```python
from build123d import *

# Parameters (mm, degrees)
EXTRUDE_1_DEPTH     = 8
CUT_EXTRUDE_1_DEPTH = 3


with BuildPart() as part:
    # Эскиз2 → Бобышка-Вытянуть1 (new body)
    with BuildSketch(Plane.XY):
        Polygon((0, 0), (40, 0), (40, 10), (27.5, 12), (27.5, 22), (42.5, 35), (42.5, 55), (-2.5, 55), (-2.5, 35), (12.5, 22), (12.5, 12), (0, 10), align=None)
    extrude(amount=EXTRUDE_1_DEPTH)

    # Эскиз3 → Вырез-Вытянуть1 (cut)
    with BuildSketch(Plane(origin=(0, 0, 0), x_dir=(-1, 0, 0), z_dir=(0, 0, -1))):
        Polygon((-40, 10), (-27.5, 12), (-27.5, 22), (-42.5, 35), (2.5, 35), (-12.5, 22), (-12.5, 12), (0, 10), align=None)
    extrude(amount=-CUT_EXTRUDE_1_DEPTH, mode=Mode.SUBTRACT)


solid = part.part
```
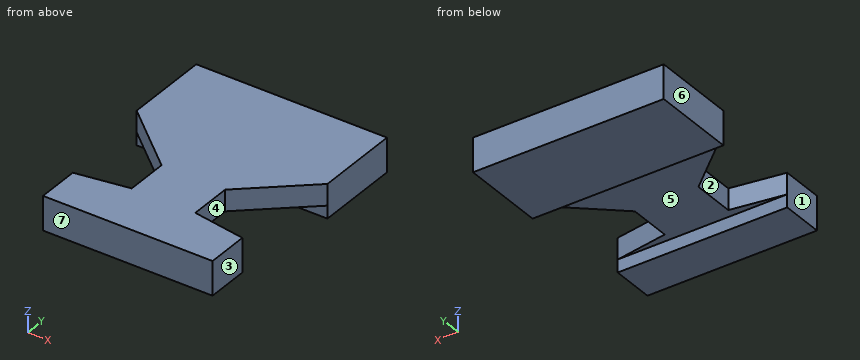
Input: part model. Units: mm. Frame: model coordinates. Face numbers are marked on the shaded views. A direction names the side the tool comes from. Coordinates: 2 decimals unless noted, no trailing zeros. Write each loop counter-clockwise with the first axis right and the second up, starting at its lowest first coordinate (ties: lowest second). Pieces come first, ordered by that corner, then holes.
1) Set-up query: the marked faces 1, 2 and 3. Return all of +Z, -Z, +X, -X, +Y, -Y with unobstructed straight access to the full face (end or side cutting, diameter ignored); none if empty.
2) Mould query, pull axis Y, two halves, no side actions, for the marked faces 4, 5, 6 and 7. Classes: pulls with the +Y half, pulls with the -Y half, needs draft (parallel to the pull), parting line crosses it, or undercut.
3) Pin query (flat end, axial travel): pin 1 Ø2.5 at (y, z) = (18.5, 6.5) entering from -X; pin 2 Ø7.5 at (x, y) = (16, 25.5) entering from -Z; pin 3 Ø3 at (y, z) = (23.5, 3.5) entering from -X. Return the tip coordinate at first contact, or that it passes through.
4) Section C-C on x = 13.5. Output: boundary loops of the cut face in (y, z), and give its area (3 significant figures).
5) Section B-B on z = 1.5. Output: boundary loops of the cut face in (x, y).
6) Material intervals for line 1 along Y through (x, z) = (37, 1.75); line 2 along Z through (x, y) = (5.5, 31.5); line 3 along Y through (x, z) = (39, 5.75), sorted ascending.
7) Section A-A on x = 30.5. Output: boundary loops of the cut face in (y, z).
8) Section D-D on z = 4.75. Output: boundary loops of the cut face in (x, y), and give its area (4 significant figures).
Check result:
1. face 1: +Z, -Z, -X, -Y
1. face 2: +Z, -Z, -X
1. face 3: +Z, -Z, +X, -Y
2. face 4: undercut
2. face 5: undercut
2. face 6: needs draft
2. face 7: pulls with the -Y half
3. pin 1: stops at x = 12.5
3. pin 2: stops at z = 3
3. pin 3: stops at x = 9.04
4. outline: (0, 0) - (10, 0) - (10, 3) - (35, 3) - (35, 0) - (55, 0) - (55, 8) - (0, 8) - close
4. area: 365 mm2
5. outline: (-2.5, 35) - (42.5, 35) - (42.5, 55) - (-2.5, 55) - close; (0, 0) - (40, 0) - (40, 10) - (0, 10) - close
6. line 1: y = 0 to 10, 35 to 55
6. line 2: z = 3 to 8
6. line 3: y = 0 to 10.16, 31.97 to 55
7. outline: (0, 0) - (10, 0) - (10, 3) - (11.52, 3) - (11.52, 8) - (0, 8) - close; (24.6, 3) - (35, 3) - (35, 0) - (55, 0) - (55, 8) - (24.6, 8) - close
8. outline: (-2.5, 35) - (12.5, 22) - (12.5, 12) - (0, 10) - (0, 0) - (40, 0) - (40, 10) - (27.5, 12) - (27.5, 22) - (42.5, 35) - (42.5, 55) - (-2.5, 55) - close
8. area: 1,895 mm2
